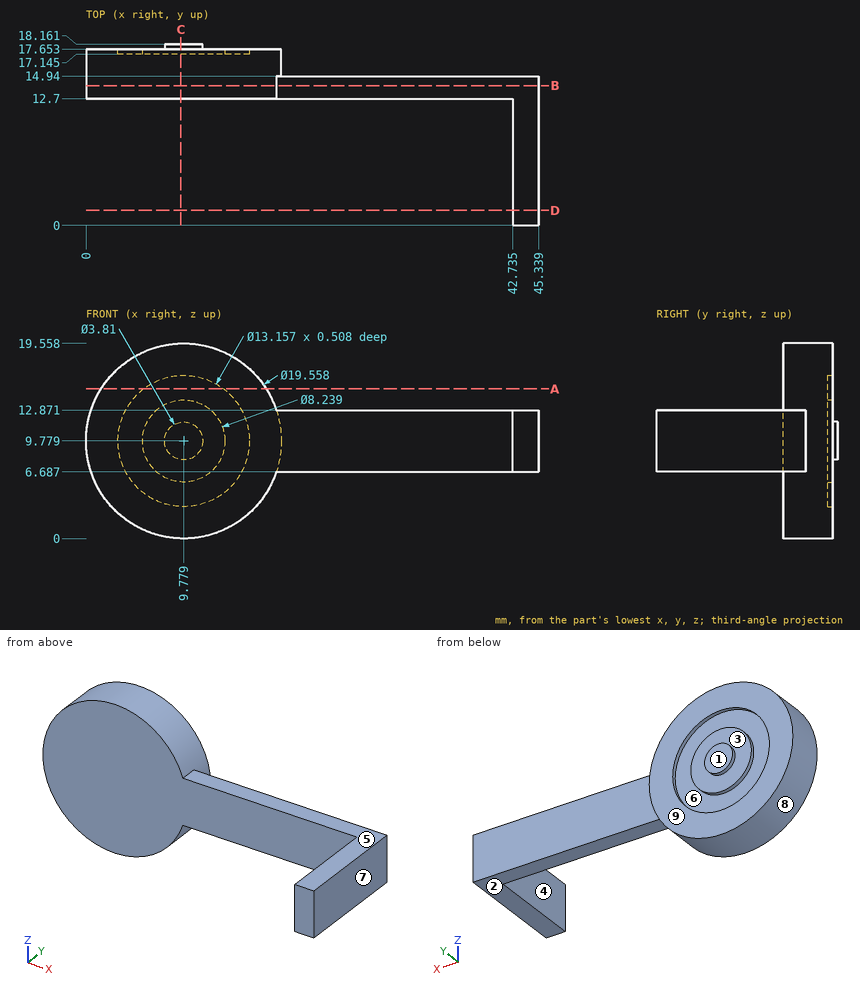
Geometry check sheet. Reference: drawing and pictorial views, mm from the part's lowest x, y, z. A direction names the side the tool comes from. Give positions to 0.01 mm unless a question says otherwise; leave off trailing zeros. Write each loop counter-clockwise with the first axis right and the second up, starting at its lowest first coordinate (ties: lowest second). Pieces come first, ordered by that corner, then holes. Notation, with made-up numbers: M -34.5,-29.75 L -14.5,-29.75 A27 cw -14.5,-4.75 Z; hole C 42.5,-20 d9. An arc over 180 degrees is marked long. Put each result on its own line as item: value. Start each with the question number.
1. Section check A-A (z = 15). Record the cut outline in (x, y) (1 decimal).
2. Draft check along X on the marked faces 6, 7, 8 and 9. Enter one of: +X half, -X half, draft (parallel to the pull), parting line (faces both ways), or undercut.
3. Section check B-B (y = 14). Record the cut outline in (x, z), and give its area (3 significant figures).
4. Set-up check for the marked faces 1, 2, 3, 4 and 5: record each of +Z, -Z, +X, -X, +Y, -Y from which the full face is reachable in a straight line by a thin tool's end or side.
5. Go/stop test with flat-tipped pins: pin 1 Ø4 at (x, y) = (10.5, 15) entering from +Z; pin 2 Ø5 at (x, z) = (37.5, 17) entering from +Y; pin 3 Ø10 at (x, z) = (22, 12.5) entering from +Y; pin 4 Ø5 at (x, z) = (35, 14.5) entering from -Y. Record where each tip stops, or that it passes through.
6. Section check C-C (x = 9.5). Record the cut outline in (y, z) (1 decimal).
7. Scan lines: line 1 along Y through (x, z) = (26, 7.5); line 2 along X through (y, z) = (16.5, 10) (1 decimal); line 3 along Y through (x, z) = (12, 5.25) (1 decimal). Record each from-to range of solid material in increasing order. Write a range as [from, to].
8. Section check D-D (y = 1.5). Record the cut outline in (x, z) (1 decimal), and give its area (3 significant figures).
Answer list:
1. outline: M 1.5,12.7 L 18,12.7 L 18,17.7 L 13.8,17.7 L 13.8,17.1 L 5.8,17.1 L 5.8,17.7 L 1.5,17.7 Z
2. face 6: undercut
2. face 7: +X half
2. face 8: parting line
2. face 9: draft
3. outline: M 19.06,6.69 L 45.34,6.69 L 45.34,12.87 L 19.06,12.87 A9.78 ccw long Z
3. area: 461 mm2
4. face 1: +Z, -Z, +X, -X, +Y
4. face 2: -Z, +X, +Y, -Y
4. face 3: +Y
4. face 4: +Z, -Z, -X, -Y
4. face 5: +Z, +X, +Y, -Y
5. pin 1: z = 19.56
5. pin 2: through
5. pin 3: y = 17.65
5. pin 4: y = 12.7
6. outline: M 12.7,0 L 17.7,0 L 17.7,3.2 L 17.1,3.2 L 17.1,5.7 L 17.7,5.7 L 17.7,7.9 L 18.2,7.9 L 18.2,11.7 L 17.7,11.7 L 17.7,13.9 L 17.1,13.9 L 17.1,16.4 L 17.7,16.4 L 17.7,19.6 L 12.7,19.6 Z
7. line 1: [12.7, 14.94]
7. line 2: [0, 19.6]
7. line 3: [12.7, 17.1]
8. outline: M 42.7,6.7 L 45.3,6.7 L 45.3,12.9 L 42.7,12.9 Z
8. area: 16.1 mm2
